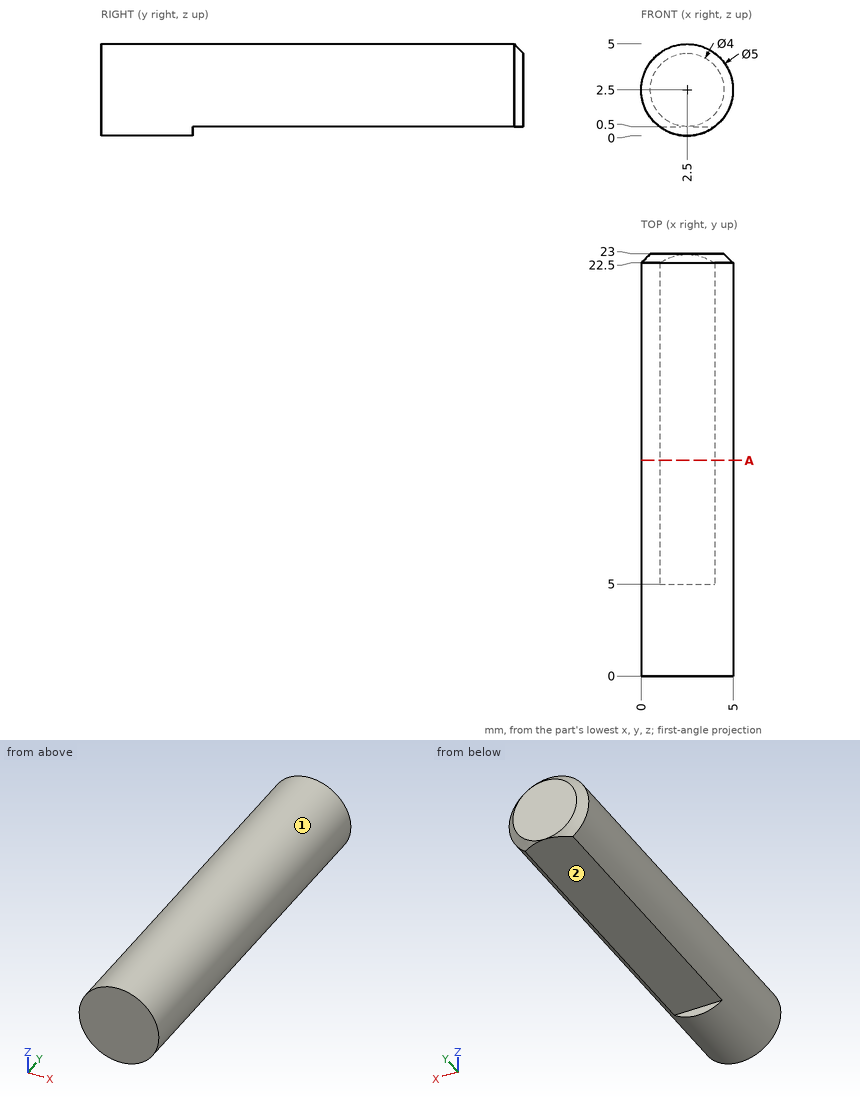
Study the drawing (mm; zero at the part's minimum x, y, z) and answer. A direction names the side the tool comes from. Round coordinates to 2 decimals unless told otherwise and drop trailing zeros. Loops run counter-clockwise (first coordinate to the right, second up) from the corner with the lowest first, then second, coordinate; pieces in that order, holes last.
Q1. Section A-A, the plane y = 11.75 is taken. Determine the outline of the cut face in (x, z), then the cut area to 3 significant figures.
Q2. Which of the six approach directions +Z, -Z, +X, -X, +Y, -Y give full straight-line access (tool end or side, diameter ignored) to the marked faces 1 and 2?
Q3. Given pin 1 Ø1 at (x, z) = (3, 4) entering from -Y; pin 2 Ø1.5 at (x, y) = (2.5, 18) entering from -Z, each flat-ended and moving along its own axis, determine where each tip first touches the part or whether it passes through.
Q4. Find the intervals of material crossed by line 1 (Z direction, x = 4.5, y = 10); line 2 (X direction, y = 15.5, z = 2.4); line 3 (Z direction, x = 2.45, y = 6.25), in increasing order.
Completed:
1. outline: (1, 0.5) - (4, 0.5) arc R2.5 ccw (long way) to start
1. area: 18.6 mm2
2. face 1: +Y, -Y
2. face 2: -Z, +X, -X, +Y
3. pin 1: stops at y = 0
3. pin 2: stops at z = 0.5
4. line 1: z = 1 to 4
4. line 2: x = 0 to 5
4. line 3: z = 0.5 to 5
